Could you check a few things on this model? Use its own coordinates, in mm. Give positions to 0.01 mm unless a question says otherwise; leave off trailing zeros. Order: outer loops, then holes, each group sorted by start corner. A loop starts at its lowest first (then second) coordinate and runs counter-clockwise, first axis right, second up. Notation, with made-up numbers: (29.25, 64.5) - (67.25, 64.5) arc R19 ccw to (67.25, 93.5) - close; hole circle Ø3 at (18, -19). An arc over 180 degrees is marked (long way). One line per question, with ' | ' between items. Start each with the question number.
1. If we mould it in two halves opening along X, with no side actions, what happens to faces 1 (the cylindrical face through (-5.158, 3.955, 2.472)), 2 (the flat face through (-3, -1, 5)), 3 (the cylindrical face through (-3, 0, 2))? For each: released by +X, released by -X, zero draft, split by the parting line, or undercut.
2. Imagine slicing it at A-A (x = 0). Please give me the cut outline in (y, z), and give its area (3 significant figures).
3. I need wall thicknesses on probe 1 along Y at (x, z) = (0, 3.15); probe 2 along Y at (x, z) = (2.5, 4.55); probe 3 along X at (y, z) = (-0.5, 1). Which ranges of each line are inside material? Lowest first, please. Write a range as from..to.
4. Imagine slicing it at C-C (z = 1.45). Please give me the cut outline in (x, y).
5. For P1, Ø1.5, axis at y = -3, z = 2, coming from the +X side; P2, Ø1.5, axis at x = -4.5, z = 0.5, coming from the -Y side; P3, Ø1.5, axis at x = -2.5, z = 1, coming from the +Y side; P4, Ø5, axis at x = 0, y = 0, coming from the +Z side, each with a flat end and sliding along its axis, tell me the tip position at first contact or that it passes through.
Autodesk Inventor part; units mm, degrees
ref_plane "YZ Plane" through (0, 0, 0) normal (1, 0, 0) x (0, 1, 0)
ref_plane "XZ Plane" through (0, 0, 0) normal (0, 1, 0) x (-1, 0, 0)
ref_plane "XY Plane" through (0, 0, 0) normal (0, 0, 1) x (1, 0, 0)
sketch "Szkic1" plane through (0, 0, 0) normal (0, 0, 1) x (1, 0, 0)
  circle A0 centre (0, 0) radius 3
  circle A1 centre (0, 0) radius 6.5
  dimension "d0" = 6
  dimension "d1" = 13
extrude "Wyciągnięcie proste1" add sketch "Szkic1" along normal blind 5
chamfer "Faza1" distance 0.5 angle 45 1 edges at (-6.5, 0, 5)
chamfer "Faza2" distance 0.5 angle 45 1 edges at (-6.5, 0, 0)
properties part number "686_bearing" material "Aluminum 6061"
Results found:
1) face 1: split by the parting line | face 2: zero draft | face 3: undercut
2) outline: (-6.5, 0.5) - (-6, 0) - (-3, 0) - (-3, 5) - (-6, 5) - (-6.5, 4.5) - close; (3, 0) - (6, 0) - (6.5, 0.5) - (6.5, 4.5) - (6, 5) - (3, 5) - close | area: 34.5 mm2
3) probe 1: y = -6.5..-3, 3..6.5 | probe 2: y = -5.95..-1.66, 1.66..5.95 | probe 3: x = -6.48..-2.96, 2.96..6.48
4) outline: circle Ø13 at (0, 0); hole circle Ø6 at (0, 0)
5) P1: stops at x = 6.1 | P2: stops at y = -5.31 | P3: stops at y = 6.26 | P4: passes through
